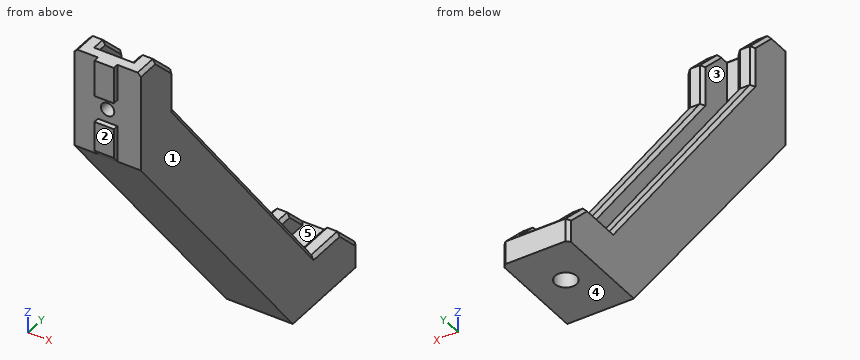
```python
from build123d import *

# Parameters (mm, degrees)
F1_DEPTH    = 10
F2_W        = 5.8
F2_H        = 30
F3_DEPTH    = 1.6
F4_W        = 5.8
F4_H        = 8
F5_DEPTH    = 1.6
F6_R        = 2
F7_DEPTH    = 15
F9_DEPTH    = 5
F10_R       = 3.25
F11_DEPTH   = 8
F13_DEPTH   = 5.8
F14_C1_SIZE = 8
F14_C2_SIZE = 8
F14_C3_SIZE = 8
F15_SIZE    = 1


with BuildPart() as f1:
    # F0 (on Right) → F1 (new body, symmetric)
    with BuildSketch(Plane.YZ):
        Polygon((70, 0), (100, 0), (100, 15), (80, 15), (15, 100), (15, 120), (0, 120), (0, 90), align=None)
    extrude(amount=F1_DEPTH, both=True)

    # F2 (on face) → F3 (join)
    with BuildSketch(Plane.XZ):
        with Locations((0, 105)):
            Rectangle(F2_W, F2_H)
    extrude(amount=F3_DEPTH)

    # F4 (on face) → F5 (cut, through all)
    with BuildSketch(Plane.XZ.offset(1.6)):
        with Locations((0, 105)):
            Rectangle(F4_W, F4_H)
    extrude(amount=-F5_DEPTH, mode=Mode.SUBTRACT)

    # F6 (on face) → F7 (cut, through all)
    with BuildSketch(Plane.XZ):
        with Locations((0, 105)):
            Circle(F6_R)
    extrude(amount=-F7_DEPTH, mode=Mode.SUBTRACT)

    # F8 (on Right) → F9 (cut, symmetric)
    with BuildSketch(Plane.YZ):
        Polygon((21.8223074079, 120), (4, 120), (4, 100), (75.5555555556, 8), (100, 8), (100, 19.4858238101), align=None)
    extrude(amount=F9_DEPTH, both=True, mode=Mode.SUBTRACT)

    # F10 (on face) → F11 (cut, through all)
    with BuildSketch(Plane.XY.offset(8)):
        with Locations((0, 86)):
            Circle(F10_R)
    extrude(amount=-F11_DEPTH, mode=Mode.SUBTRACT)

    # F12 (on face) → F13 (cut, through all)
    with BuildSketch(Plane.YZ.offset(2.9)):
        Polygon((-1.6, 90), (0, 90), (-1.6, 92.0571428571), align=None)
    extrude(amount=-F13_DEPTH, mode=Mode.SUBTRACT)

    # F14: chamfer of 8 on 4 edges, made by hand

    # F14_c1
    f14_c1_edges = [f1.edges().sort_by_distance(p)[0] for p in [
        (7.5, 100, 15),
    ]]
    chamfer(f14_c1_edges, length=F14_C1_SIZE)

    # F14_c2
    f14_c2_edges = [f1.edges().sort_by_distance(p)[0] for p in [
        (-7.5, 15, 120),
    ]]
    chamfer(f14_c2_edges, length=F14_C2_SIZE)

    # F14_c3
    f14_c3_edges = [f1.edges().sort_by_distance(p)[0] for p in [
        (7.5, 15, 120),
    ]]
    chamfer(f14_c3_edges, length=F14_C3_SIZE)

    # F15
    f15_edges = [f1.edges().sort_by_distance(p)[0] for p in [
        (10, 47.5, 57.5),
        (5, 47.5, 57.5),
        (10, 15, 106),
        (5, 15, 106),
        (-5, 15, 106),
        (-10, 15, 106),
        (-5, 47.5, 57.5),
        (-10, 47.5, 57.5),
        (10, 86, 15),
        (5, 86, 15),
        (-5, 86, 15),
        (-10, 86, 15),
        (-10, 100, 3.5),
        (10, 100, 3.5),
        (10, 3.5, 120),
        (5, 5.5, 120),
        (-5, 5.5, 120),
        (-10, 3.5, 120),
        (0, 4, 120),
        (5, 39.777778, 54),
        (-5, 39.777778, 54),
        (10, 96, 11),
        (5, 95.5, 11.5),
        (-5, 95.5, 11.5),
        (-10, 96, 11),
        (10, 11, 116),
        (5, 11, 116),
        (-5, 11, 116),
        (-10, 11, 116),
    ]]
    chamfer(f15_edges, length=F15_SIZE)


solid = f1.part
```
The listing builds one solid part. Answer for the finished solid, in the listing's coordinates (mm). Face numbers are marked on the shaded views. A direction names the side the tool comes from. Coordinates: 2 decimals unless noted, no trailing zeros. Loops run counter-clockwise (first coordinate to the right, second up) from the corner with the lowest first, then second, coordinate; pieces in that order, holes last. Notation, with made-up numbers: (-19.75, -23.5) -> (4.25, -23.5) arc R15 ccw to (4.25, -8.5) -> close; hole circle Ø3 at (16, 28.5). An arc over 180 degrees is marked (long way). Return JSON: item names as keys, results as strings. Group by question number.
(1) Find the intervals of material crossed by probe 1 along Z at (x, y) = (0.5, 77); probe 2 along X at (y, z) = (75, 10); probe 3 along Y at (x, z) = (0, 2.25), in increasing order. Write a range as from..to.
(2) A cutting plane is placed at D-D on x = -7.5. Write down the section's boundary in (y, z).
(3) A cutting plane is placed at B-B on y = 86. Write down the section's boundary in (x, z).
(4) A cutting plane is placed at A-A on x = 0. Write down the section's boundary in (y, z), and give its area (3 significant figures).
(5) Determine the mould class of the marked faces 1, 2 and 3 for opening direction X: released by +X, released by -X, zero draft, split by the parting line, or undercut.
(6) A cutting plane is placed at C-C on z = 105. Write down the section's boundary in (x, y), and give its area (3 significant figures).
(7) Given pin 1 Ø1.8 at (y, z) = (-0.5, 96.5) entering from -X; pin 2 Ø2.5 at (x, z) = (-7.5, 104.5) entering from +Y; pin 3 Ø2 at (x, z) = (4.5, 65.5) entering from -Y; pin 4 Ø1 at (x, z) = (-7.5, 90) entering from +Y, each flat-ended and moving along its own axis, determine where each tip first touches the part or whether it passes through.
(8) Which of the six approach directions +Z, -Z, +X, -X, +Y, -Y give full straight-line access (tool end or side, diameter ignored) to the marked faces 4 and 5?
The answers:
{
 "1": {"probe 1": "z = 0..8", "probe 2": "x = -10..-4.79, 4.79..10", "probe 3": "y = 68.25..82.75, 89.25..100"},
 "2": {"outline": "(0, 90) -> (70, 0) -> (100, 0) -> (100, 7) -> (92, 15) -> (80, 15) -> (15, 100) -> (15, 112) -> (7, 120) -> (0, 120) -> close"},
 "3": {"outline": "(-10, 0) -> (-3.25, 0) -> (-3.25, 8) -> (-5, 8) -> (-5, 14) -> (-6, 15) -> (-9, 15) -> (-10, 14) -> close; (3.25, 0) -> (10, 0) -> (10, 14) -> (9, 15) -> (6, 15) -> (5, 14) -> (5, 8) -> (3.25, 8) -> close"},
 "4": {"outline": "(-1.6, 92.06) -> (70, 0) -> (82.75, 0) -> (82.75, 8) -> (75.56, 8) -> (4, 100) -> (4, 103) -> (0, 103) -> (0, 101) -> (-1.6, 101) -> close; (-1.6, 109) -> (0, 109) -> (0, 107) -> (4, 107) -> (4, 119) -> (3, 120) -> (-1.6, 120) -> close; (89.25, 0) -> (100, 0) -> (100, 7) -> (99, 8) -> (89.25, 8) -> close", "area": "1,350 mm^2"},
 "5": {"face 1": "released by +X", "face 2": "zero draft", "face 3": "undercut"},
 "6": {"outline": "(-10, 0) -> (-2, 0) -> (-2, 4) -> (-5, 4) -> (-5, 14) -> (-6, 15) -> (-9, 15) -> (-10, 14) -> close; (2, 0) -> (10, 0) -> (10, 14) -> (9, 15) -> (6, 15) -> (5, 14) -> (5, 4) -> (2, 4) -> close", "area": "172 mm^2"},
 "7": {"pin 1": "stops at x = -10", "pin 2": "stops at y = 15", "pin 3": "stops at y = 18.28", "pin 4": "stops at y = 23.03"},
 "8": {"face 4": "-Z, +X, -X, +Y, -Y", "face 5": "+Z, +Y"}
}
